Build history of the part. All positions in model axes, mm. Face numbers are marked on the shaded views. A direction names the side the tool comes from. Coordinates: 2 decimals unless noted, no trailing zeros. Write each loop counter-clockwise with the first axis right and the second up, starting at its lowest first coordinate (ties: lowest second). Pieces come first, ordered by that corner, then holes.
Autodesk Fusion 360 part; units mm, degrees
sketch "Sketch1" plane through (0, 0, 0) normal (0, 0, 1) x (1, 0, 0)
  circle A0 centre (0, 0) radius 3.25
  dimension "d1" = 6.5
extrude "Extrude1" add sketch "Sketch1" along normal blind 1
sketch "Sketch2" plane through (0, 0, 1) normal (0, 0, 1) x (-1, 0, 0)
  circle A0 centre (0, 0) radius 3.25
  circle A1 centre (0, 0) radius 2.25
  dimension "d4" = 4.5
extrude "Extrude2" add sketch "Sketch2" along normal blind 2.5 contours A1
fillet "Fillet1" radius 0.5 1 edges at (2.0977, 0.8136, 3.5)
fillet "Fillet2" radius 0.125 1 edges at (-3.0301, -1.1753, 1)
sketch "Sketch3" plane through (0, 0, 0) normal (0, 0, 1) x (1, 0, 0)
  circle A0 centre (0, 0) radius 1.25
  dimension "d11" = 2.5
extrude "Extrude3" cut sketch "Sketch3" along normal blind 0.5
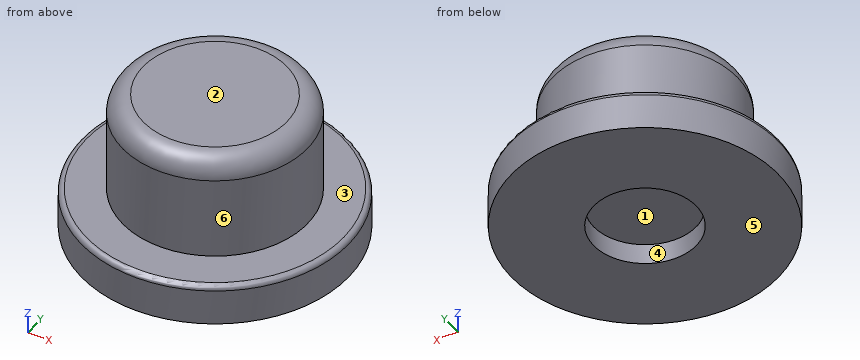
1. 3-axis set-ups, long thin cutter, end or side, ignore diameter. For the marked faces 1, 2 and 3: which of +Z, -Z, +X, -X, +Y, -Y reach the whole face in a straight line?
Computed values:
face 1: -Z
face 2: +Z, +X, -X, +Y, -Y
face 3: +Z
2. Saw through at A-A on y = 0. List the corners of the cut face in (x, z) (3 decimals), plus the area to 3 significant figures.
Computed values:
outline: (-3.25, 0) - (-1.25, 0) - (-1.25, 0.5) - (1.25, 0.5) - (1.25, 0) - (3.25, 0) - (3.25, 0.875) arc R0.125 ccw to (3.125, 1) - (2.25, 1) - (2.25, 3) arc R0.5 ccw to (1.75, 3.5) - (-1.75, 3.5) arc R0.5 ccw to (-2.25, 3) - (-2.25, 1) - (-3.125, 1) arc R0.125 ccw to (-3.25, 0.875) - close
area: 16.4 mm2
3. Probe line 1 along Y through (x, z) = (-3, 0.6); line 2 along Z through (x, y) = (0.25, 0.75); line 3 along Y through (x, z) = (0, 0.1). List the from-to ranges inside material, lowest first.
Computed values:
line 1: y = -1.25 to 1.25
line 2: z = 0.5 to 3.5
line 3: y = -3.25 to -1.25, 1.25 to 3.25
4. Saw through at D-D on z = 1.2. List the corners of the cut face in (x, y), plus the area to 3 significant figures.
Computed values:
outline: circle Ø4.5 at (0, 0)
area: 15.9 mm2
5. Mould opens along Y. For the marked faces 4, 5 and 6 say: +Y half, -Y half, draft (parallel to the pull), parting line (faces both ways), or undercut.
Computed values:
face 4: undercut
face 5: draft
face 6: parting line
6. Flat gauge pins, fed straight in: pin 1 (2 mm diameter, centred on x = -2, z = 3, fed in from -Y); pin 2 (2 mm diameter, centred on x = 2, z = 0.5, fed in from -Y); pin 3 (0.8 mm diameter, centred on x = 0, y = -0.5, fed in from -Z). Where does each tip first touch, or does it go through?
Computed values:
pin 1: stops at y = -2.02
pin 2: stops at y = -3.09
pin 3: stops at z = 0.5
7. Saw through at C-C on z = 0.6. List the corners of the cut face in (x, y), plus the area to 3 significant figures.
Computed values:
outline: circle Ø6.5 at (0, 0)
area: 33.2 mm2
